Geometry: final body of the model. Coordinates: model frame, mm. A direction names the side the tool comes from. Give positions to 0.01 mm unless a question says otherwise; leave off trailing zeros. Loops run counter-clockwise (first coordinate to the right, second up) from the corner with the lowest first, then second, coordinate; pieces in that order, holes last.
```python
from build123d import *

# Parameters (mm, degrees)
BOSS_EXTRUDE1_DEPTH = 3
SKETCH2_R           = 1.6
CUT_EXTRUDE1_DEPTH  = 37.458880948
SKETCH3_R           = 3.2
CUT_EXTRUDE2_DEPTH  = 2.3
CUT_EXTRUDE3_DEPTH  = 2
FILLET1_R           = 2


with BuildPart() as part:
    # Sketch1 → Boss-Extrude1 (new body)
    with BuildSketch(Plane.XY):
        with BuildLine():
            Line((-10, -30), (10, -30))
            Line((10, -30), (10, -4.671400751))
            ThreePointArc((10, -4.671400751), (11.868024086, 1.148476201), (16.774193548, 4.794019088))
            ThreePointArc((16.774193548, 4.794019088), (20.5, 10), (16.774193548, 15.205980912))
            ThreePointArc((16.774193548, 15.205980912), (11.868024086, 18.851523799), (10, 24.671400751))
            Line((10, 24.671400751), (10, 30))
            Line((10, 30), (-10, 30))
            Line((-10, 30), (-10, 24.671400751))
            ThreePointArc((-10, 24.671400751), (-11.868024086, 18.851523799), (-16.774193548, 15.205980912))
            ThreePointArc((-16.774193548, 15.205980912), (-20.5, 10), (-16.774193548, 4.794019088))
            ThreePointArc((-16.774193548, 4.794019088), (-11.868024086, 1.148476201), (-10, -4.671400751))
            Line((-10, -4.671400751), (-10, -30))
        make_face()
    extrude(amount=BOSS_EXTRUDE1_DEPTH)

    # Sketch2 → Cut-Extrude1 (cut, through all)
    with BuildSketch(Plane.XY.offset(3)):
        with Locations((-15, 10)):
            Circle(SKETCH2_R)
        with Locations((15, 10)):
            Circle(SKETCH2_R)
        with BuildLine():
            Line((-3.65, 26.9), (-3.65, -26.9))
            ThreePointArc((-3.65, -26.9), (-4.75, -28), (-5.85, -26.9))
            Line((-5.85, -26.9), (-5.85, 26.9))
            ThreePointArc((-5.85, 26.9), (-4.75, 28), (-3.65, 26.9))
        make_face()
        with BuildLine():
            Line((5.85, 26.9), (5.85, -26.9))
            ThreePointArc((5.85, -26.9), (4.75, -28), (3.65, -26.9))
            Line((3.65, -26.9), (3.65, 26.9))
            ThreePointArc((3.65, 26.9), (4.75, 28), (5.85, 26.9))
        make_face()
    extrude(amount=-CUT_EXTRUDE1_DEPTH, mode=Mode.SUBTRACT)

    # Sketch3 → Cut-Extrude2 (cut)
    with BuildSketch(Plane.XY.offset(3)):
        with Locations((-15, 10)):
            Circle(SKETCH3_R)
        with Locations((15, 10)):
            Circle(SKETCH3_R)
    extrude(amount=-CUT_EXTRUDE2_DEPTH, mode=Mode.SUBTRACT)

    # Sketch4 → Cut-Extrude3 (cut)
    with BuildSketch(Plane(origin=(0, 0, 0), x_dir=(-1, 0, 0), z_dir=(0, 0, -1))):
        with BuildLine():
            Line((-2.65, 26.9), (-2.65, -26.9))
            ThreePointArc((-2.65, -26.9), (-4.75, -29), (-6.85, -26.9))
            Line((-6.85, -26.9), (-6.85, 26.9))
            ThreePointArc((-6.85, 26.9), (-4.75, 29), (-2.65, 26.9))
        make_face()
        with BuildLine():
            Line((2.65, -26.9), (2.65, 26.9))
            ThreePointArc((2.65, 26.9), (4.75, 29), (6.85, 26.9))
            Line((6.85, 26.9), (6.85, -26.9))
            ThreePointArc((6.85, -26.9), (4.75, -29), (2.65, -26.9))
        make_face()
    extrude(amount=-CUT_EXTRUDE3_DEPTH, mode=Mode.SUBTRACT)

    # Fillet1
    fillet1_edges = [part.edges().sort_by_distance(p)[0] for p in [
        (10, -30, 1.5),
        (-10, -30, 1.5),
        (-10, 30, 1.5),
        (10, 30, 1.5),
    ]]
    fillet(fillet1_edges, radius=FILLET1_R)


solid = part.part
```
Q1. Reachability of faces 1 (the face through (10, 26, 1)), 2 (the face through (4.8, -28, 2.5)), 3 (the face through (-6, 0, 2)) from +Z, -Z, +X, -X, +Y, -Y: full face, straight path, thin tool, end or side. Return the list, or none.
Q2. Section query A-A, the plane y = -10.5. Return loops of the section in (x, z).
Q3. Section query D-D, the plane y = 18. Return loops of the section in (x, z).
Q4. Mould query, pull axis Y, two halves, no side actions, for faces 4 (the face through (-10, -16, 1)), 5 (the face through (-13.6, 8.6, 0.7)), 6 (the face through (9.4, -29.43, 1.52)). Classes: +Y half, -Y half, draft (parallel to the pull), parting line (faces both ways), or undercut.
Q5. Material intervals for probe 1 along X at (y, z) = (-21, 1.2); probe 2 along X at (y, z) = (-7, 2.95); probe 3 along X at (y, z) = (9, 1.65), sorted ascending.
Q6. Section query B-B, the plane z = 1.5. Return loops of the section in (x, y), and give its area (3 significant figures).
Q7. Section query C-C, the plane x = -4.75. Return loops of the section in (y, z).
Q8. Pin query (flat end, axial travel): pin 1 Ø3.5 at (x, y) = (15, 10) entering from +Z; pin 2 Ø1 at (y, z) = (-3.5, 1) entering from +X; pin 3 Ø0.8 at (y, z) = (6.5, 2.5) entering from -X. Return the tip coordinate at first contact, or that it passes through.
Resolved:
1. face 1: +Z, -Z, +X, +Y
1. face 2: +Z, -Z
1. face 3: -Z
2. outline: (-10, 0) - (-6.85, 0) - (-6.85, 2) - (-5.85, 2) - (-5.85, 3) - (-10, 3) - close; (-3.65, 2) - (-2.65, 2) - (-2.65, 0) - (2.65, 0) - (2.65, 2) - (3.65, 2) - (3.65, 3) - (-3.65, 3) - close; (5.85, 2) - (6.85, 2) - (6.85, 0) - (10, 0) - (10, 3) - (5.85, 3) - close
3. outline: (-12.55, 0) - (-6.85, 0) - (-6.85, 2) - (-5.85, 2) - (-5.85, 3) - (-12.55, 3) - close; (-3.65, 2) - (-2.65, 2) - (-2.65, 0) - (2.65, 0) - (2.65, 2) - (3.65, 2) - (3.65, 3) - (-3.65, 3) - close; (5.85, 2) - (6.85, 2) - (6.85, 0) - (12.55, 0) - (12.55, 3) - (5.85, 3) - close
4. face 4: draft
4. face 5: undercut
4. face 6: -Y half
5. probe 1: x = -10 to -6.85, -2.65 to 2.65, 6.85 to 10
5. probe 2: x = -10 to -5.85, -3.65 to 3.65, 5.85 to 10
5. probe 3: x = -20.41 to -18.04, -11.96 to -6.85, -2.65 to 2.65, 6.85 to 11.96, 18.04 to 20.41
6. outline: (-16.77, 4.79) arc R10 cw to (-10, -4.67) - (-10, -28) arc R2 ccw to (-8, -30) - (8, -30) arc R2 ccw to (10, -28) - (10, -4.67) arc R10 cw to (16.77, 4.79) arc R5.5 ccw to (16.77, 15.21) arc R10 cw to (10, 24.67) - (10, 28) arc R2 ccw to (8, 30) - (-8, 30) arc R2 ccw to (-10, 28) - (-10, 24.67) arc R10 cw to (-16.77, 15.21) arc R5.5 ccw to start; hole circle Ø6.4 at (-15, 10); hole (-6.85, -26.9) arc R2.1 ccw to (-2.65, -26.9) - (-2.65, 26.9) arc R2.1 ccw to (-6.85, 26.9) - close; hole (2.65, -26.9) arc R2.1 ccw to (6.85, -26.9) - (6.85, 26.9) arc R2.1 ccw to (2.65, 26.9) - close; hole circle Ø6.4 at (15, 10)
6. area: 919 mm2
7. outline: (-30, 0) - (-29, 0) - (-29, 2) - (-28, 2) - (-28, 3) - (-30, 3) - close; (28, 2) - (29, 2) - (29, 0) - (30, 0) - (30, 3) - (28, 3) - close
8. pin 1: stops at z = 0.7
8. pin 2: stops at x = 10.14
8. pin 3: stops at x = -19.54
